```python
from build123d import *

# Parameters (mm, degrees)
SKETCH1_R           = 35
SKETCH1_R_2         = 2.1
BOSS_EXTRUDE1_DEPTH = 10
SKETCH2_W           = 140
SKETCH2_H           = 10
BOSS_EXTRUDE2_DEPTH = 48
SKETCH3_R           = 3.85
CUT_EXTRUDE1_DEPTH  = 2.3


with BuildPart() as part:
    # Sketch1 → Boss-Extrude1 (new body)
    with BuildSketch(Plane.XY):
        with BuildLine():
            Line((0, -64.1), (-70, -64.1))
            Line((-70, -64.1), (-59.369947745, 8.672329831))
            ThreePointArc((-59.369947745, 8.672329831), (0, 60), (59.369947745, 8.672329831))
            Line((59.369947745, 8.672329831), (70, -64.1))
            Line((70, -64.1), (0, -64.1))
        make_face()
        Circle(SKETCH1_R, mode=Mode.SUBTRACT)
        with Locations((-50, 0)):
            Circle(SKETCH1_R_2, mode=Mode.SUBTRACT)
        with Locations((-43.301270189, 25)):
            Circle(SKETCH1_R_2, mode=Mode.SUBTRACT)
        with Locations((-25, 43.301270189)):
            Circle(SKETCH1_R_2, mode=Mode.SUBTRACT)
        with Locations((0, 50)):
            Circle(SKETCH1_R_2, mode=Mode.SUBTRACT)
        with Locations((25, 43.301270189)):
            Circle(SKETCH1_R_2, mode=Mode.SUBTRACT)
        with Locations((43.301270189, 25)):
            Circle(SKETCH1_R_2, mode=Mode.SUBTRACT)
        with Locations((50, 0)):
            Circle(SKETCH1_R_2, mode=Mode.SUBTRACT)
        with Locations((43.301270189, -25)):
            Circle(SKETCH1_R_2, mode=Mode.SUBTRACT)
        with Locations((25, -43.301270189)):
            Circle(SKETCH1_R_2, mode=Mode.SUBTRACT)
        with Locations((0, -50)):
            Circle(SKETCH1_R_2, mode=Mode.SUBTRACT)
        with Locations((-25, -43.301270189)):
            Circle(SKETCH1_R_2, mode=Mode.SUBTRACT)
        with Locations((-43.301270189, -25)):
            Circle(SKETCH1_R_2, mode=Mode.SUBTRACT)
    extrude(amount=BOSS_EXTRUDE1_DEPTH)

    # Sketch2 → Boss-Extrude2 (add)
    with BuildSketch(Plane.XY.offset(10)):
        with Locations((0, -69.1)):
            Rectangle(SKETCH2_W, SKETCH2_H)
    extrude(amount=-BOSS_EXTRUDE2_DEPTH)

    # Sketch3 → Cut-Extrude1 (cut)
    with BuildSketch(Plane.XY.offset(10)):
        with Locations((0, -50)):
            Circle(SKETCH3_R)
        with Locations((-25, -43.301270189)):
            Circle(SKETCH3_R)
        with Locations((-43.301270189, -25)):
            Circle(SKETCH3_R)
        with Locations((-50, 0)):
            Circle(SKETCH3_R)
        with Locations((-43.301270189, 25)):
            Circle(SKETCH3_R)
        with Locations((-25, 43.301270189)):
            Circle(SKETCH3_R)
        with Locations((0, 50)):
            Circle(SKETCH3_R)
        with Locations((25, 43.301270189)):
            Circle(SKETCH3_R)
        with Locations((43.301270189, 25)):
            Circle(SKETCH3_R)
        with Locations((50, 0)):
            Circle(SKETCH3_R)
        with Locations((43.301270189, -25)):
            Circle(SKETCH3_R)
        with Locations((25, -43.301270189)):
            Circle(SKETCH3_R)
    extrude(amount=-CUT_EXTRUDE1_DEPTH, mode=Mode.SUBTRACT)


solid = part.part
```
Check sheet for the modelled part. Datum: model origin and axes. Units: mm. A direction names the side the tool comes from. Coordinates: 2 decimals unless noted, no trailing zeros. Order: outer loops, then holes, each group sorted by start corner. A loop starts at its lowest first (then second) coordinate and runs counter-clockwise, first axis right, second up. Notation, with made-up numbers: (32.5, 1.5) -> (68.5, 1.5) arc R23 cw to (68.5, 9.5) -> close; hole circle Ø1 at (28, -27). An arc over 180 degrees is marked (long way). Write each question's results on one line, items separated by ' | '. Start each with the question number.
1) Set-up check for faces 3 (the face through (-1, -64.1, -19)), 4 (the face through (45, -27, 7.7)), 5 (the face through (-0.46, -52.05, 3.8)): record each of +Z, -Z, +X, -X, +Y, -Y from which the full face is reachable in a straight line by a thin tool's end or side.
2) Depth check by flat-ended pin: pin 1 (2.5 mm diameter, centred on x = -52, y = -0.5, fed in from +Z); pin 2 (10 mm diameter, centred on x = 33.5, y = 30, fed in from -Z); pin 3 (2.5 mm diameter, centred on x = 25, y = 43.3, fed in from +Z); pin 4 (3 mm diameter, centred on x = -27.5, z = -16, fed in from +Y). Enter the tip coordinate at first touch or a pass-through.
3) Section check C-C (x = -50). Enter the section's corners in (y, z), and give its area (3 significant figures).
4) Material ranges on line 1 along Y through (x, z) = (-44, 4); line 2 along X through (y, z) = (-25, 6); line 3 along X through (y, z) = (25, 2.75), recorded low to high.
5) Section check A-A (x = 0). Enter the section's corners in (y, z), and give its area (3 significant figures).
6) Section check B-B (y = -32). Enter the section's corners in (x, z), and give its area (3 significant figures).
7) Section check D-D (y = 25). Enter the section's corners in (x, z).
8) Draft check along X on faces 1 (the face through (-1, -36, 10)), 2 (the face through (24.5, 47.12, 8.87)). Enter one of: pulls with the +X half, pulls with the -X half, needs draft (parallel to the pull), parting line crosses it, or undercut.
Checked values:
1) face 3: -Z, +X, -X, +Y | face 4: +Z | face 5: +Z, -Z
2) pin 1: z = 7.7 | pin 2: z = 0 | pin 3: through | pin 4: y = -64.1
3) outline: (-74.1, -38) -> (-64.1, -38) -> (-64.1, 0) -> (-2.1, 0) -> (-2.1, 7.7) -> (-3.85, 7.7) -> (-3.85, 10) -> (-74.1, 10) -> close; (2.1, 0) -> (33.17, 0) -> (33.17, 10) -> (3.85, 10) -> (3.85, 7.7) -> (2.1, 7.7) -> close | area: 1,400 mm²
4) line 1: -74.1 to -26.98, -23.02 to 23.02, 26.98 to 40.79 | line 2: -64.29 to -45.4, -41.2 to -24.49, 24.49 to 41.2, 45.4 to 64.29 | line 3: -54.54 to -45.4, -41.2 to -24.49, 24.49 to 41.2, 45.4 to 54.54
5) outline: (-74.1, -38) -> (-64.1, -38) -> (-64.1, 0) -> (-52.1, 0) -> (-52.1, 7.7) -> (-53.85, 7.7) -> (-53.85, 10) -> (-74.1, 10) -> close; (-47.9, 0) -> (-35, 0) -> (-35, 10) -> (-46.15, 10) -> (-46.15, 7.7) -> (-47.9, 7.7) -> close; (35, 0) -> (47.9, 0) -> (47.9, 7.7) -> (46.15, 7.7) -> (46.15, 10) -> (35, 10) -> close; (52.1, 0) -> (60, 0) -> (60, 10) -> (53.85, 10) -> (53.85, 7.7) -> (52.1, 7.7) -> close | area: 921 mm²
6) outline: (-65.31, 0) -> (-14.18, 0) -> (-14.18, 10) -> (-65.31, 10) -> close; (14.18, 0) -> (65.31, 0) -> (65.31, 10) -> (14.18, 10) -> close | area: 1,020 mm²
7) outline: (-54.54, 0) -> (-45.4, 0) -> (-45.4, 7.7) -> (-47.15, 7.7) -> (-47.15, 10) -> (-54.54, 10) -> close; (-41.2, 0) -> (-24.49, 0) -> (-24.49, 10) -> (-39.45, 10) -> (-39.45, 7.7) -> (-41.2, 7.7) -> close; (24.49, 0) -> (41.2, 0) -> (41.2, 7.7) -> (39.45, 7.7) -> (39.45, 10) -> (24.49, 10) -> close; (45.4, 0) -> (54.54, 0) -> (54.54, 10) -> (47.15, 10) -> (47.15, 7.7) -> (45.4, 7.7) -> close
8) face 1: needs draft | face 2: undercut
